```python
from build123d import *

# Parameters (mm, degrees)
F1_DEPTH       = 40
F2_R           = 5
F4_D           = 3.3
F4_DEPTH       = 13.5
F4_CSINK_D     = 6.72
F4_CSINK_ANGLE = 90
F4_TIP         = 0.9914200214


with BuildPart() as f1:
    # F0 (on Front) → F1 (new body)
    with BuildSketch(Plane.XZ):
        with BuildLine():
            Line((-40, -2.5), (-22.360679775, -2.5))
            ThreePointArc((-22.360679775, -2.5), (-22.5, 0), (-22.360679775, 2.5))
            Line((-22.360679775, 2.5), (-40, 2.5))
            Line((-40, 2.5), (-40, -2.5))
        make_face()
        with BuildLine():
            ThreePointArc((-22.360679775, 2.5), (-22.5, 0), (-22.360679775, -2.5))
            Line((-22.360679775, -2.5), (-17.3205080757, -2.5))
            ThreePointArc((-17.3205080757, -2.5), (-17.5, 0), (-17.3205080757, 2.5))
            Line((-17.3205080757, 2.5), (-22.360679775, 2.5))
        make_face()
        with BuildLine():
            Line((17.3205080757, 2.5), (22.360679775, 2.5))
            ThreePointArc((22.360679775, 2.5), (0, 22.5), (-22.360679775, 2.5))
            Line((-22.360679775, 2.5), (-17.3205080757, 2.5))
            ThreePointArc((-17.3205080757, 2.5), (0, 17.5), (17.3205080757, 2.5))
        make_face()
        with BuildLine():
            Line((17.3205080757, -2.5), (22.360679775, -2.5))
            ThreePointArc((22.360679775, -2.5), (22.4651429434, -1.2519395078), (22.5, 0))
            ThreePointArc((22.5, 0), (22.4651429434, 1.2519395078), (22.360679775, 2.5))
            Line((22.360679775, 2.5), (17.3205080757, 2.5))
            ThreePointArc((17.3205080757, 2.5), (17.4550693399, 1.2532175939), (17.5, 0))
            ThreePointArc((17.5, 0), (17.4550693399, -1.2532175939), (17.3205080757, -2.5))
        make_face()
        with BuildLine():
            Line((22.360679775, -2.5), (40, -2.5))
            Line((40, -2.5), (40, 2.5))
            Line((40, 2.5), (22.360679775, 2.5))
            ThreePointArc((22.360679775, 2.5), (22.4651429434, 1.2519395078), (22.5, 0))
            ThreePointArc((22.5, 0), (22.4651429434, -1.2519395078), (22.360679775, -2.5))
        make_face()
    extrude(amount=F1_DEPTH)

    # F2
    f2_edges = [f1.edges().sort_by_distance(p)[0] for p in [
        (-40, -40, 0),
        (-40, 0, 0),
        (40, -40, 0),
        (40, 0, 0),
    ]]
    fillet(f2_edges, radius=F2_R)

    # F4
    with Locations(Plane.XY.offset(2.5)):
        with Locations((-31.6543355584, -9.2338668182), (-31.5996408463, -31.6989757121), (31.2322638929, -8.5554420948), (31.6695906222, -31.6989757121)):
            CounterSinkHole(F4_D / 2, F4_CSINK_D / 2, depth=F4_DEPTH, counter_sink_angle=F4_CSINK_ANGLE)
            with Locations((0, 0, -(F4_DEPTH + F4_TIP / 2))):  # 118° drill point
                Cone(0, F4_D / 2, F4_TIP, mode=Mode.SUBTRACT)


solid = f1.part
```
The listing builds one solid part. Answer for the finished solid, in the listing's coordinates (mm). A direction names the side the tool comes from. Round coordinates to 2 decimals unless told otherwise and drop trailing zeros. Loops run counter-clockwise (first coordinate to the right, second up) from the corner with the lowest first, then second, coordinate; pieces in that order, holes last.
1) A cutting plane is placed at A-A on y = -14. Determine the outline of the cut face in (x, z), plus the area to 3 significant figures.
Outcome:
outline: (-40, -2.5) - (-17.32, -2.5) arc R17.5 cw (long way) to (17.32, -2.5) - (40, -2.5) - (40, 2.5) - (22.36, 2.5) arc R22.5 ccw to (-22.36, 2.5) - (-40, 2.5) - close
area: 515 mm2
2) For a pull along Y with two mould halves and no side action, classify faces 1 (the face through (39, -38, 0)), 2 (the face through (29, -20, -2.5)), 3 (the face through (30.096, -31.203, -0.878)), 4 (the face through (39, -2, 0)) as released by +Y, released by -Y, zero draft, split by the parting line, or undercut.
Outcome:
face 1: released by -Y
face 2: zero draft
face 3: undercut
face 4: released by +Y
3) For faces 5 (the face through (-39, -38, 0)), 6 (the face through (-31, -20, 2.5)), 7 (the face through (31, -20, 2.5)), determine the directions among +Z, -Z, +X, -X, +Y, -Y from which every point of the face is accessible in a straight line to the end or side of a thin tool.
Outcome:
face 5: +Z, -Z, -X, -Y
face 6: +Z, -X, +Y, -Y
face 7: +Z, +X, +Y, -Y
4) Given P1, Ø1.5, axis at y = -23.5, z = 12.5, coming from the +X side; P2, Ø1, axis at x = -8.5, y = -5.5, coming from the -Z side; P3, Ø4.5, axis at x = 31.23, y = -8.56, coming from the +Z side; P4, Ø2.5, axis at x = -31.65, y = -9.23, coming from the -Z side, each flat-ended and moving along its own axis, determine where each tip first touches the part or whether it passes through.
Outcome:
P1: stops at x = 19.19
P2: stops at z = 15.01
P3: stops at z = 1.4
P4: passes through
5) Consider line 1 (Z direction, x = 34.5, y = -34); line 2 (X direction, y = -26.5, z = -0.5); line 3 (X direction, y = -28.5, z = 15.5). Determine where each line is inside the solid, lowest interval first.
Outcome:
line 1: z = -2.5 to 2.5
line 2: x = -40 to -17.49, 17.49 to 40
line 3: x = -16.31 to -8.12, 8.12 to 16.31
6) A cutting plane is placed at D-D on x = 19. Determine the outline of the cut face in (y, z), plus the area to 3 significant figures.
Outcome:
outline: (-40, -2.5) - (0, -2.5) - (0, 12.05) - (-40, 12.05) - close
area: 582 mm2
7) A cutting plane is placed at B-B on z = 8.25. Determine the outline of the cut face in (x, y), plus the area to 3 significant figures.
Outcome:
outline: (-20.93, -40) - (-15.43, -40) - (-15.43, 0) - (-20.93, 0) - close; (15.43, -40) - (20.93, -40) - (20.93, 0) - (15.43, 0) - close
area: 440 mm2
8) A cutting plane is placed at C-C on z = 16.25. Determine the outline of the cut face in (x, y).
Outcome:
outline: (-15.56, -40) - (-6.5, -40) - (-6.5, 0) - (-15.56, 0) - close; (6.5, -40) - (15.56, -40) - (15.56, 0) - (6.5, 0) - close
